Autodesk Inventor part; units mm, degrees
ref_plane "Work Plane1" through (0, 0, 0) normal (-0.9848, 0, -0.1736) x (0, 1, 0)
ref_plane "Work Plane2" through (14.7721, 0, 2.6047) normal (-0.9848, 0, -0.1736) x (0, 1, 0)
ref_plane "YZ Plane" through (0, 0, 0) normal (1, 0, 0) x (0, 1, 0)
sketch "Sketch1" plane through (0, 0, 0) normal (0, 1, 0) x (-1, 0, 0)
  line L0 (-17, 0) -> (17, 0)
  line L1 (17, 0) -> (17, -75)
  line L2 (17, -75) -> (-17, -75)
  line L3 (-17, -58) -> (-17, 0)
  arc A0 (-17, -58) -> (17, -58) centre (0, -58) ccw
  line L4 (23.8, 0) -> (-23.8, 0)
  point P0 (0, 0)
  point P1 (0, 0)
  dimension "d0" = 34
  dimension "d1" = 75
  dimension "d2" = 34
revolve "Revolution1" add sketch "Sketch1" angle 360 about axis through (-10, 0, 0) along (1, 0, 0) contours L0 L1 A0 L3
sketch "Sketch2" plane through (17, 0, 0) normal (1, 0, 0) x (0, 0, -1)
  circle A0 centre (0, 0) radius 58
  circle A1 centre (0, 0) radius 22.5
  dimension "d4" = 45
extrude "Extrusion1" cut sketch "Sketch2" against normal blind 14
sketch "Sketch3" plane through (17, 0, 0) normal (1, 0, 0) x (0, 0, -1)
  circle A0 centre (0, 0) radius 6.5
  dimension "d7" = 13
extrude "Extrusion2" cut sketch "Sketch3" against normal blind 20
ref_plane "Work Plane1" through (0, 0, 0) normal (-0.9848, 0, -0.1736) x (0, 1, 0)
ref_plane "Work Plane2" through (14.7721, 0, 2.6047) normal (-0.9848, 0, -0.1736) x (0, 1, 0)
sketch "Sketch6" plane through (3, 0, 0) normal (1, 0, 0) x (0, 0, -1)
  circle A0 centre (0, 0) radius 58
  circle A1 centre (0, 0) radius 22.5
  line L0 (-54.9704, -18.5) -> (-54.9704, 18.5)
  line L1 (-19.8997, -10.5) -> (-19.8997, 10.5)
  circle A2 centre (0, 0) radius 22.5
  circle A3 centre (0, 0) radius 58
  line L2 (-19.8997, 10.5) -> (-54.9704, 18.5)
  line L3 (-19.8997, -10.5) -> (-54.9704, -18.5)
  dimension "d20" = 37
  dimension "d21" = 21
extrude "Extrusion4" add sketch "Sketch6" along normal up to surface contours L0 A0 | L2 A1 L3 L0 surface through (14.7721, 0, 2.6047) normal (-0.9848, 0, -0.1736)
pattern_circular "Circular Pattern1" count 4 over 360 about axis through (-10, 0, 0) along (1, 0, 0) of "Extrusion4"
mirror "Mirror1" about plane through (0, 0, 0) normal (1, 0, 0) of "Extrusion1", "Extrusion2", "Extrusion4", "Circular Pattern1"
ref_plane "Work Plane3" through (0, 0, 0) normal (1, 0, 0) x (0, 1, 0)
properties part number "Llanta" material "Acetal Resin, Black"
Input: part model. Units: mm. Frame: model coordinates. A direction names the side the tool comes from. Give positions to 0.01 mm unless a question says otherwise; leave off trailing zeros. Loops run counter-clockwise (first coordinate to the right, second up) from the corner with the lowest first, then second, coordinate; pieces in that order, holes last.
1) Reachability of faces 3 (the flat face through (3, -32, -32)), 4 (the flat face through (-3, -32, -28)), 5 (the cylindrical face through (-0.238, 3.955, 5.158)) from +Z, -Z, +X, -X, +Y, -Y: full face, straight path, thin tool, end or side. Return the list, or none.
A:
face 3: +X
face 4: -X
face 5: +X, -X
2) Contact query for flat-ended pins moving along their axis: pin 1 (3 mm diameter, centred on x = 9, y = 0.5, fed in from -Z); pin 2 (6 mm diameter, centred on x = -4.5, y = 9.5, fed in from -Z); pin 3 (6 mm diameter, centred on y = -42, z = -33, fed in from +X); pin 4 (10.5 mm diameter, centred on y = 0, z = 0, fed in from -X). Output: stop coordinate, or through.
A:
pin 1: stops at z = -73.25
pin 2: stops at z = -74.47
pin 3: stops at x = 3
pin 4: passes through
3) Section query A-A on z = 0. Return the cut outline in (x, y), and give its area (3 significant figures).
A:
outline: (-17, -58) arc R17 ccw to (17, -58) - (5, -58) - (11.26, -22.5) - (17, -22.5) - (17, -6.5) - (-17, -6.5) - (-17, -22.5) - (-11.26, -22.5) - (-5, -58) - close; (-17, 6.5) - (17, 6.5) - (17, 22.5) - (11.26, 22.5) - (5, 58) - (17, 58) arc R17 ccw to (-17, 58) - (-5, 58) - (-11.26, 22.5) - (-17, 22.5) - close
area: 3,150 mm2
4) Mould query, pull axis Z, two halves, no side actions, for faces 1 (the flat face through (8.316, -39.217, -0.259)), 2 (the flat face through (-3, 28, 32)). Classes: released by +Z, released by -Z, zero draft, split by the parting line, or undercut.
A:
face 1: undercut
face 2: undercut
5) Line query: L1, parallel to Y at x = 9, z = -28; L2, parallel to Y at x = 9, z = 30.5; L3, parallel to Y at x = 12.5, z = -2. Output: solid intervals per line, ascending.
A:
L1: y = -66.79 to -50.79, -12.35 to 12.35, 50.79 to 66.79
L2: y = -65.69 to -49.33, -12.92 to 12.92, 49.33 to 65.69
L3: y = -69.49 to -57.97, -22.41 to -6.18, 6.18 to 22.41, 57.97 to 69.49
